Source: CAD feature listing. Evaluate the final solid. Frame: model axes, mm. A direction names the side the tool comes from. Give positions to 0.01 mm unless a question says otherwise; leave off trailing zeros. Loops run counter-clockwise (first coordinate to the right, second up) from the corner with the lowest first, then second, coordinate; pieces in that order, holes last. Notation, with made-up numbers: M -38,81 L -26,81 A33 cw -26,111 Z; hole C -40,-8.75 d4. An arc over 180 degrees is marked long. Answer in a Markdown table with one row per item.
```python
from build123d import *

# Parameters (mm, degrees)
SKETCH1_W           = 5
SKETCH1_H           = 5
SKETCH1_R           = 0.935
BOSS_EXTRUDE3_DEPTH = 3
FILLET3_R           = 2
BOSS_EXTRUDE4_DEPTH = 9
FILLET5_R           = 0.5
SKETCH6_R           = 2.5
BOSS_EXTRUDE5_DEPTH = 4.35
FILLET6_R           = 0.5


with BuildPart() as part:
    # Sketch1 → Boss-Extrude3 (new body)
    with BuildSketch(Plane.XY):
        Rectangle(SKETCH1_W, SKETCH1_H)
        Circle(SKETCH1_R, mode=Mode.SUBTRACT)
    extrude(amount=BOSS_EXTRUDE3_DEPTH)

    # Fillet3
    fillet3_edges = [part.edges().sort_by_distance(p)[0] for p in [
        (-2.5, 2.5, 1.5),
        (2.5, 2.5, 1.5),
    ]]
    fillet(fillet3_edges, radius=FILLET3_R)

    # Sketch3 → Boss-Extrude4 (add)
    with BuildSketch(Plane.XZ.offset(2.5)):
        with BuildLine():
            ThreePointArc((0, 2.471779521), (-1, 1.471779521), (0, 0.471779521))
            Line((0, 0.471779521), (0, 2.471779521))
        make_face()
        with BuildLine():
            Line((0, 2.471779521), (0, 0.471779521))
            ThreePointArc((0, 0.471779521), (0.707106781, 0.76467274), (1, 1.471779521))
            ThreePointArc((1, 1.471779521), (0.707106781, 2.178886302), (0, 2.471779521))
        make_face()
    extrude(amount=BOSS_EXTRUDE4_DEPTH)

    # Fillet5
    fillet5_edges = [part.edges().sort_by_distance(p)[0] for p in [
        (0, -2.5, 0.471779521),
    ]]
    fillet(fillet5_edges, radius=FILLET5_R)

    # Sketch6 → Boss-Extrude5 (add)
    with BuildSketch(Plane.XZ.offset(11.5)):
        with Locations((0, 1.471779521)):
            Circle(SKETCH6_R)
    extrude(amount=BOSS_EXTRUDE5_DEPTH)

    # Fillet6
    fillet6_edges = [part.edges().sort_by_distance(p)[0] for p in [
        (0, -11.5, 0.471779521),
    ]]
    fillet(fillet6_edges, radius=FILLET6_R)


solid = part.part
```
Q1. Section query B-B (z = 0.25). Give the number of separate pieces and of enclosed holes in the cut face, plus the area to 3 significant figures.
Values follow:
| item | result |
|---|---|
| separate pieces | 2 |
| enclosed holes | 1 |
| area | 39.7 mm^2 |
Q2. Section query D-D (z = 3.2). Output: boundary loops of the cut face in (x, y).
Values follow:
| item | result |
|---|---|
| outline | M -1.81,-15.85 L 1.81,-15.85 L 1.81,-11.5 L -1.81,-11.5 Z |
Q3. Section query A-A (y = 0). Output: boundary loops of the cut face in (x, z) (3 decimals).
Values follow:
| item | result |
|---|---|
| outline | M -2.5,0 L -0.935,0 L -0.935,3 L -2.5,3 Z; M 0.935,0 L 2.5,0 L 2.5,3 L 0.935,3 Z |
Q4. Mould query, pull axis Y, two halves, no side actions, for faces 1 (the cylindrical face through (1.9, 1.93, 1.52)), 2 (the flat face through (-2, -2.5, 1)), 3 (the flat face through (0, -15.85, 2)). Classes: +Y half, -Y half, draft (parallel to the pull), parting line (faces both ways), or undercut.
Values follow:
| item | result |
|---|---|
| face 1 | +Y half |
| face 2 | undercut |
| face 3 | -Y half |
Q5. Section query C-C (y = -14.5). Output: boundary loops of the cut face in (x, z).
Values follow:
| item | result |
|---|---|
| outline | C 0,1.47 d5 |
Q6. Contact query for flat-ended pins moving along their axis: pin 1 Ø1 at (y, z) = (-6, 0.5) entering from -X; pin 2 Ø2.5 at (x, y) = (0.5, 1) entering from +Z; pin 3 Ø1.1 at (x, y) = (0, 0) entering from -Z; pin 4 Ø1.5 at (x, y) = (-1, -0.5) entering from -Z. Output: stop coordinate, or through.
Values follow:
| item | result |
|---|---|
| pin 1 | x = -0.88 |
| pin 2 | z = 3 |
| pin 3 | through |
| pin 4 | z = 0 |
Q7. Ray query, probe 1 along Y at (x, z) = (0, 1.65) (3 decimals); probe 2 along Z at (x, y) = (1.2, 1.25); probe 3 along Y at (x, z) = (-0.5, -0.05). Return the intervals inside material, ascending. Write a range as from..to.
Values follow:
| item | result |
|---|---|
| probe 1 | -15.85..-0.935, 0.935..2.5 |
| probe 2 | 0..3 |
| probe 3 | -15.85..-11.5 |
Q8. Reachability of faces 4 (the cylindrical face through (-0.54, -13.64, -0.97)), 5 (the flat face through (0, -1.1, 3)), 6 (the flat face through (0, -1.1, 0)) from +Z, -Z, +X, -X, +Y, -Y: full face, straight path, thin tool, end or side. Return the list, or none.
Values follow:
| item | result |
|---|---|
| face 4 | -Y |
| face 5 | +Z, +X, -X, +Y |
| face 6 | -Z, +X, -X, +Y |
